from build123d import *

# Parameters (mm, degrees)
BASE_PROFILE_W              = 76.2
BASE_PROFILE_H              = 76.2
BASE_DEPTH                  = 2
CONNECTOR_PROFILE_R         = 2.5
CONNECTOR_BODY_DEPTH        = 7.5
HEAD_PROFILE_R              = 3
CONNECTOR_HEAD_DEPTH        = 2.6
CONNECTOR_HEAD_CHAMFER_SIZE = 0.65
CONNECTOR_GAP_REACH         = 57.696
TRIM_START                  = -2.6
TRIM_HEAD_DEPTH             = 2.39107
ROUND_EDGE_R                = 5


with BuildPart() as part:
    # Base Profile → Base (new, symmetric)
    with BuildSketch(Plane(origin=(0, 0, 0), x_dir=(1, 0, 0), z_dir=(0, 1, 0))):
        Rectangle(BASE_PROFILE_W, BASE_PROFILE_H)
    extrude(amount=BASE_DEPTH, both=True)

    # Connector Profile → Connector Body (add)
    with BuildSketch(Plane(origin=(0, 2, 0), x_dir=(1, 0, 0), z_dir=(0, 1, 0))):
        with Locations(Location((-21.59, 21.59, 0), (0, 0, 90))):
            Circle(CONNECTOR_PROFILE_R)
        with Locations(Location((9.302081056, -9.302081056, 0), (0, 0, 90))):
            Circle(CONNECTOR_PROFILE_R)
    extrude(amount=CONNECTOR_BODY_DEPTH)

    # Head Profile → Connector Head (add)
    with BuildSketch(Plane(origin=(0, 9.5, 0), x_dir=(1, 0, 0), z_dir=(0, 1, 0))):
        with Locations(Location((-21.59, 21.59, 0), (0, 0, 270))):
            Circle(HEAD_PROFILE_R)
        with Locations(Location((9.302081056, -9.302081056, 0), (0, 0, 270))):
            Circle(HEAD_PROFILE_R)
    extrude(amount=CONNECTOR_HEAD_DEPTH)

    # Connector Head Chamfer
    connector_head_chamfer_edges = [part.edges().sort_by_distance(p)[0] for p in [
        (-21.59, 12.1, -24.59),
        (9.302081056, 12.1, 6.302081056),
    ]]
    chamfer(connector_head_chamfer_edges, length=CONNECTOR_HEAD_CHAMFER_SIZE)

    # Connector Gap: up to this face of the body (flat: up to its plane)
    connector_gap_end = Plane(part.part.faces().sort_by_distance((0.041835549, 2, 0.041835549))[0])
    # Gap Profile → Connector Gap (cut, up to the picked face)
    with BuildSketch(Plane(origin=(0, 12.1, 0), x_dir=(1, 0, 0), z_dir=(0, 1, 0)), mode=Mode.PRIVATE) as connector_gap_sk1:
        with BuildLine():
            Line((-22.24, 24.518736929), (-22.24, 18.661263071))
            ThreePointArc((-22.24, 18.661263071), (-21.59, 18.59), (-20.94, 18.661263071))
            Line((-20.94, 18.661263071), (-20.94, 24.518736929))
            ThreePointArc((-20.94, 24.518736929), (-21.59, 24.59), (-22.24, 24.518736929))
        make_face()
    connector_gap_tool1 = split(extrude(connector_gap_sk1.sketch, amount=-CONNECTOR_GAP_REACH, mode=Mode.PRIVATE), bisect_by=connector_gap_end, keep=Keep.BOTH, mode=Mode.PRIVATE)
    # Gap Profile → Connector Gap (cut, up to the picked face)
    with BuildSketch(Plane(origin=(0, 12.1, 0), x_dir=(1, 0, 0), z_dir=(0, 1, 0)), mode=Mode.PRIVATE) as connector_gap_sk2:
        with BuildLine():
            Line((8.652081056, -6.373344127), (8.652081056, -12.230817986))
            ThreePointArc((8.652081056, -12.230817986), (9.302081056, -12.302081056), (9.952081056, -12.230817986))
            Line((9.952081056, -12.230817986), (9.952081056, -6.373344127))
            ThreePointArc((9.952081056, -6.373344127), (9.302081056, -6.302081056), (8.652081056, -6.373344127))
        make_face()
    connector_gap_tool2 = split(extrude(connector_gap_sk2.sketch, amount=-CONNECTOR_GAP_REACH, mode=Mode.PRIVATE), bisect_by=connector_gap_end, keep=Keep.BOTH, mode=Mode.PRIVATE)
    add(connector_gap_tool1.solids().sort_by(Axis((-21.59, 12.1, -21.59), (0, -1, 0)))[0], mode=Mode.SUBTRACT)
    add(connector_gap_tool2.solids().sort_by(Axis((9.302081, 12.1, 9.302081), (0, -1, 0)))[0], mode=Mode.SUBTRACT)

    # Trim Profile → Trim Head (cut)
    with BuildSketch(Plane(origin=(0, 12.1, 0), x_dir=(1, 0, 0), z_dir=(0, 1, 0)).offset(TRIM_START)):
        with BuildLine():
            Line((7.606682873, -6.827081056), (10.99747924, -6.827081056))
            ThreePointArc((10.99747924, -6.827081056), (9.302081056, -6.302081056), (7.606682873, -6.827081056))
        make_face()
        with BuildLine():
            Line((7.606682873, -11.777081056), (10.99747924, -11.777081056))
            ThreePointArc((10.99747924, -11.777081056), (9.302081056, -12.302081056), (7.606682873, -11.777081056))
        make_face()
        with BuildLine():
            Line((-23.285398183, 24.065), (-19.894601817, 24.065))
            ThreePointArc((-19.894601817, 24.065), (-21.59, 24.59), (-23.285398183, 24.065))
        make_face()
        with BuildLine():
            Line((-23.285398183, 19.115), (-19.894601817, 19.115))
            ThreePointArc((-19.894601817, 19.115), (-21.59, 18.59), (-23.285398183, 19.115))
        make_face()
    extrude(amount=TRIM_HEAD_DEPTH, mode=Mode.SUBTRACT)

    # Round Edge
    round_edge_edges = [part.edges().sort_by_distance(p)[0] for p in [
        (38.1, 0, 38.1),
        (-38.1, 0, 38.1),
        (-38.1, 0, -38.1),
        (38.1, 0, -38.1),
    ]]
    fillet(round_edge_edges, radius=ROUND_EDGE_R)


solid = part.part
Could you check a few things on this model? Use its own coordinates, in mm. A direction names the side the tool comes from. Give positions to 0.01 mm unless a question says otherwise; leave off trailing zeros. Order: outer loops, then holes, each group sorted by start corner. A loop starts at its lowest first (then second) coordinate and runs counter-clockwise, first axis right, second up. Notation, with made-up numbers: (43.5, 32.5) - (101.5, 32.5) arc R17 cw to (101.5, 47.5) - close; hole circle Ø5 at (-11, 54). An arc over 180 degrees is marked (long way). One line per item, written item: value. Start each with the question number.
1. For faces 1 (the face through (-24.59, 10.46, -21.63)), 2 (the face through (-19.09, 5.7, -21.54)), 3 (the face through (8.652, 7, 9)), 4 (the face through (-18.59, 10.46, -21.55)), which set-ups out of +Z, -Z, +X, -X, +Y, -Y let a thin tool reach every point of the face, with its end or its side?
2. Imagine slicing it at C-C on x = 25.5. List the corners of the cut face in (y, z) for me.
3. If I drill on probe 1 along Y at (x, z) = (23, 28.5), over which ranges is the centre line in solid material (lowest first)?
4. Thinking about a two-plate mould opening in Y: for faces 5 (the face through (11.83, 11.92, 9.35)), 6 (the face through (36.67, -0.03, -36.6)), 7 (the face through (-24.09, 5.7, -21.64)), which applies, +Y half, -Y half, draft (parallel to the pull), parting line (faces both ways), or undercut?
5. Imagine slicing it at B-B on z = 25. List the corners of the cut face in (x, y) for me.
6. For P1, Ø1, axis at x = -17, y = 8, coming from the -Z side; P2, Ø2.5, axis at y = 7.5, z = -20.5, coming from the -X side; P3, Ø0.8, axis at x = 10.5, y = 11, coming from the -Z side; P4, Ø2.5, axis at y = 7.5, z = 10, coming from the +X side, each with a flat end and sliding along its axis, tell me the tip position at first contact or that it passes through.
7. Imagine slicing it at A-A on y = 7.5. List the corners of the cut face in (x, z) for me.
Values:
1. face 1: -X, +Y
1. face 2: +X
1. face 3: +Z, -Z, +Y
1. face 4: +X, +Y
2. outline: (-2, -38.1) - (2, -38.1) - (2, 38.1) - (-2, 38.1) - close
3. probe 1: -2 to 2
4. face 5: +Y half
4. face 6: draft
4. face 7: undercut
5. outline: (-38.1, -2) - (38.1, -2) - (38.1, 2) - (-38.1, 2) - close
6. P1: through
6. P2: x = -24.09
6. P3: z = 6.83
6. P4: x = 11.8
7. outline: (-22.24, -24) - (-22.24, -19.18) arc R2.5 ccw to start; (-20.94, -24) arc R2.5 ccw to (-20.94, -19.18) - close; (8.65, 6.89) - (8.65, 11.72) arc R2.5 ccw to start; (9.95, 6.89) arc R2.5 ccw to (9.95, 11.72) - close
